```python
from build123d import *

# Parameters (mm, degrees)
SKETCH1_W                 = 17.4625
SKETCH1_H                 = 11.90625
BOSS_EXTRUDE1_DEPTH       = 25.4
SKETCH2_W                 = 3.175
SKETCH2_H                 = 5.55625
CUT_EXTRUDE1_DEPTH        = 25.4
SKETCH4_R                 = 2.286
CUT_EXTRUDE2_DEPTH        = 25.4
F_8_32_TAPPED_HOLE1_D     = 3.4544
F_8_32_TAPPED_HOLE1_DEPTH = 11.1125
F_8_32_TAPPED_HOLE1_TIP   = 1.037806461


with BuildPart() as part:
    # Sketch1 → Boss-Extrude1 (new body)
    with BuildSketch(Plane(origin=(0, 0, 0), x_dir=(1, 0, 0), z_dir=(0, 1, 0))):
        with Locations((8.73125, 5.953125)):
            Rectangle(SKETCH1_W, SKETCH1_H)
    extrude(amount=BOSS_EXTRUDE1_DEPTH)

    # Sketch2 → Cut-Extrude1 (cut)
    with BuildSketch(Plane.XY):
        Polygon((0, 15.08125), (6.35, 15.08125), (9.525, 15.08125), (9.525, 25.4), (0, 25.4), align=None)
        with Locations((7.9375, 12.303125)):
            Rectangle(SKETCH2_W, SKETCH2_H)
    extrude(amount=-CUT_EXTRUDE1_DEPTH, mode=Mode.SUBTRACT)

    # Sketch4 → Cut-Extrude2 (cut)
    with BuildSketch(Plane.ZY):
        with Locations((-5.953125, 6.35)):
            Circle(SKETCH4_R)
    extrude(amount=-CUT_EXTRUDE2_DEPTH, mode=Mode.SUBTRACT)

    # #8-32 Tapped Hole1
    with Locations(Plane(origin=(0, 25.4, 0), x_dir=(1, 0, 0), z_dir=(0, 1, 0))):
        with Locations((13.843, 6.35)):
            Hole(F_8_32_TAPPED_HOLE1_D / 2, depth=F_8_32_TAPPED_HOLE1_DEPTH)
            with Locations((0, 0, -(F_8_32_TAPPED_HOLE1_DEPTH + F_8_32_TAPPED_HOLE1_TIP / 2))):  # 118° drill point
                Cone(0, F_8_32_TAPPED_HOLE1_D / 2, F_8_32_TAPPED_HOLE1_TIP, mode=Mode.SUBTRACT)


solid = part.part
```
The listing builds one solid part. Answer for the finished solid, in the listing's coordinates (mm). A direction names the side the tool comes from. Give positions to 0.01 mm unless a question says otherwise; leave off trailing zeros. Loops run counter-clockwise (first coordinate to the right, second up) from the corner with the lowest first, then second, coordinate; pieces in that order, holes last. Notation, with made-up numbers: (61, 78) - (112, 78) arc R18 ccw to (112, 112) - close; hole circle Ø3 at (20, 3). An arc over 180 degrees is marked (long way). Return JSON: item names as keys, results as strings. Group by question number.
1. Determine the mould class of faces 5 (the flat face through (8, 9.525, -6)), 6 (the cylindrical face through (8.609, 6.451, -8.237)), 7 (the flat face through (11, 10, 0)) for opening direction Z: pulls with the +Z half, pulls with the -Z half, needs draft (parallel to the pull), parting line crosses it, or undercut.
2. Straight lines are drawn through the part: line 1 (Y direction, x = 11.75, z = -6); line 2 (X direction, y = 17, z = -6.35) (1 decimal); line 3 (Y direction, x = 4.75, z = -8.75). For each, find the intervals that lie inside material, in ascending order. Write a range as [from, to].
3. Given pin 1 Ø2 at (x, z) = (13.843, -6.35) entering from +Y; pin 2 Ø5 at (y, z) = (19, -9) entering from -X (3 decimals); pin 3 Ø5 at (x, z) = (3.5, -4.5) entering from +Y, each flat-ended and moving along its own axis, determine where each tip first touches the part or whether it passes through.
4. Which of the six approach directions +Z, -Z, +X, -X, +Y, -Y give full straight-line access (tool end or side, diameter ignored) to faces 1 (the cylindrical face through (15.57, 19.77, -6.43)), 2 (the flat face through (17.462, 13, -6)), 3 (the flat face through (6.35, 12, -6)), 4 (the flat face through (3, 15.081, -6))?
5. Find section B-B (x = 6.75). Write down the section's boundary in (y, z) (3 decimals).
Verdict:
{
 "1": {"face 5": "needs draft", "face 6": "undercut", "face 7": "pulls with the +Z half"},
 "2": {"line 1": "y = [0, 4.06], [8.64, 25.4]", "line 2": "x = [9.5, 12.1], [15.6, 17.5]", "line 3": "y = [0, 15.08]"},
 "3": {"pin 1": "stops at y = 13.85", "pin 2": "stops at x = 9.525", "pin 3": "stops at y = 15.08"},
 "4": {"face 1": "+Y", "face 2": "+Z, -Z, +X, +Y, -Y", "face 3": "+Z, -Z, +Y", "face 4": "+Z, -Z, -X, +Y"},
 "5": {"outline": "(0, -11.906) - (9.525, -11.906) - (9.525, 0) - (0, 0) - close; hole circle Ø4.572 at (6.35, -5.953)"}
}
